```python
from build123d import *

# Parameters (mm, degrees)
F1_DEPTH      = 50.8
F1_DEPTH_BACK = 50.8


with BuildPart() as f1:
    # F0 (on Right) → F1 (new body, two sides)
    with BuildSketch(Plane.YZ) as f1_sk:
        with BuildLine():
            Line((-33.213852, 0), (0, 0))
            Line((0, 0), (39.494485, 0))
            Line((39.494485, 0), (39.494485, 0.787258))
            ThreePointArc((39.494485, 0.787258), (39.42009, 0.966864), (39.240485, 1.041258))
            Line((39.240485, 1.041258), (38.534891, 1.041258))
            ThreePointArc((38.534891, 1.041258), (38.355286, 1.115653), (38.280891, 1.295258))
            Line((38.280891, 1.295258), (38.280891, 1.323207))
            ThreePointArc((38.280891, 1.323207), (38.206496, 1.502813), (38.026891, 1.577207))
            Line((38.026891, 1.577207), (36.921442, 1.577207))
            ThreePointArc((36.921442, 1.577207), (36.739611, 1.653856), (36.667521, 1.837542))
            Line((36.667521, 1.837542), (36.67292, 2.053964))
            Line((36.67292, 2.053964), (36.67292, 10.407829))
            ThreePointArc((36.67292, 10.407829), (36.52413, 10.767039), (36.16492, 10.915829))
            Line((36.16492, 10.915829), (35.66636, 10.915829))
            ThreePointArc((35.66636, 10.915829), (35.529192, 10.956051), (35.435466, 11.063979))
            Line((35.435466, 11.063979), (34.805344, 12.438487))
            ThreePointArc((34.805344, 12.438487), (34.711619, 12.546415), (34.57445, 12.586637))
            Line((34.57445, 12.586637), (33.903744, 12.586637))
            ThreePointArc((33.903744, 12.586637), (33.752842, 12.536952), (33.660976, 12.407335))
            Line((33.660976, 12.407335), (32.40961, 8.340397))
            ThreePointArc((32.40961, 8.340397), (32.317744, 8.21078), (32.166843, 8.161095))
            Line((32.166843, 8.161095), (28.181681, 8.161095))
            Line((28.181681, 8.161095), (28.181681, 8.340397))
            Line((28.181681, 8.340397), (27.995555, 8.340397))
            Line((27.995555, 8.340397), (27.995555, 8.161095))
            Line((27.995555, 8.161095), (24.103897, 8.161095))
            Line((24.103897, 8.161095), (24.103897, 8.339632))
            Line((24.103897, 8.339632), (23.922047, 8.339632))
            Line((23.922047, 8.339632), (23.922047, 8.161095))
            Line((23.922047, 8.161095), (20.075496, 8.161095))
            Line((20.075496, 8.161095), (20.075496, 8.348511))
            Line((20.075496, 8.348511), (19.897439, 8.348511))
            Line((19.897439, 8.348511), (19.897439, 8.161095))
            Line((19.897439, 8.161095), (16.041223, 8.161095))
            Line((16.041223, 8.161095), (16.041223, 8.341497))
            Line((16.041223, 8.341497), (15.859049, 8.341497))
            Line((15.859049, 8.341497), (15.859049, 8.161095))
            Line((15.859049, 8.161095), (11.9808, 8.161095))
            Line((11.9808, 8.161095), (11.9808, 8.331576))
            Line((11.9808, 8.331576), (11.798942, 8.331576))
            Line((11.798942, 8.331576), (11.798942, 8.161095))
            Line((11.798942, 8.161095), (7.925448, 8.161095))
            Line((7.925448, 8.161095), (7.925448, 8.35035))
            Line((7.925448, 8.35035), (7.742784, 8.35035))
            Line((7.742784, 8.35035), (7.742784, 8.161095))
            Line((7.742784, 8.161095), (3.581181, 8.161095))
            ThreePointArc((3.581181, 8.161095), (3.444013, 8.201317), (3.350287, 8.309245))
            Line((3.350287, 8.309245), (1.457299, 12.438487))
            ThreePointArc((1.457299, 12.438487), (1.363573, 12.546415), (1.226405, 12.586637))
            Line((1.226405, 12.586637), (0, 12.586637))
            Line((0, 12.586637), (-1.226405, 12.586637))
            ThreePointArc((-1.226405, 12.586637), (-1.363573, 12.546415), (-1.457299, 12.438487))
            Line((-1.457299, 12.438487), (-3.350287, 8.309245))
            ThreePointArc((-3.350287, 8.309245), (-3.444013, 8.201317), (-3.581181, 8.161095))
            Line((-3.581181, 8.161095), (-7.742784, 8.161095))
            Line((-7.742784, 8.161095), (-7.742784, 8.35035))
            Line((-7.742784, 8.35035), (-7.925448, 8.35035))
            Line((-7.925448, 8.35035), (-7.925448, 8.161095))
            Line((-7.925448, 8.161095), (-11.798942, 8.161095))
            Line((-11.798942, 8.161095), (-11.798942, 8.331576))
            Line((-11.798942, 8.331576), (-11.9808, 8.331576))
            Line((-11.9808, 8.331576), (-11.9808, 8.161095))
            Line((-11.9808, 8.161095), (-15.859049, 8.161095))
            Line((-15.859049, 8.161095), (-15.859049, 8.341497))
            Line((-15.859049, 8.341497), (-16.041223, 8.341497))
            Line((-16.041223, 8.341497), (-16.041223, 8.161095))
            Line((-16.041223, 8.161095), (-19.897439, 8.161095))
            Line((-19.897439, 8.161095), (-19.897439, 8.348511))
            Line((-19.897439, 8.348511), (-20.075496, 8.348511))
            Line((-20.075496, 8.348511), (-20.075496, 8.161095))
            Line((-20.075496, 8.161095), (-23.922047, 8.161095))
            Line((-23.922047, 8.161095), (-23.922047, 8.339632))
            Line((-23.922047, 8.339632), (-24.103897, 8.339632))
            Line((-24.103897, 8.339632), (-24.103897, 8.161095))
            Line((-24.103897, 8.161095), (-27.995555, 8.161095))
            Line((-27.995555, 8.161095), (-27.995555, 8.340397))
            Line((-27.995555, 8.340397), (-28.181681, 8.340397))
            Line((-28.181681, 8.340397), (-28.181681, 8.161095))
            Line((-28.181681, 8.161095), (-32.166843, 8.161095))
            ThreePointArc((-32.166843, 8.161095), (-32.317744, 8.21078), (-32.40961, 8.340397))
            Line((-32.40961, 8.340397), (-33.660976, 12.407335))
            ThreePointArc((-33.660976, 12.407335), (-33.752842, 12.536952), (-33.903744, 12.586637))
            Line((-33.903744, 12.586637), (-34.57445, 12.586637))
            ThreePointArc((-34.57445, 12.586637), (-34.711619, 12.546415), (-34.805344, 12.438487))
            Line((-34.805344, 12.438487), (-35.435466, 11.063979))
            ThreePointArc((-35.435466, 11.063979), (-35.529192, 10.956051), (-35.66636, 10.915829))
            Line((-35.66636, 10.915829), (-36.16492, 10.915829))
            ThreePointArc((-36.16492, 10.915829), (-36.52413, 10.767039), (-36.67292, 10.407829))
            Line((-36.67292, 10.407829), (-36.67292, 2.053964))
            ThreePointArc((-36.67292, 2.053964), (-36.52413, 1.694754), (-36.16492, 1.545964))
            Line((-36.16492, 1.545964), (-34.873612, 1.545964))
            ThreePointArc((-34.873612, 1.545964), (-34.694007, 1.47157), (-34.619612, 1.291964))
            Line((-34.619612, 1.291964), (-34.619612, 1.104801))
            ThreePointArc((-34.619612, 1.104801), (-34.545217, 0.925196), (-34.365612, 0.850801))
            Line((-34.365612, 0.850801), (-33.721852, 0.850801))
            ThreePointArc((-33.721852, 0.850801), (-33.542246, 0.776406), (-33.467852, 0.596801))
            Line((-33.467852, 0.596801), (-33.467852, 0.254))
            ThreePointArc((-33.467852, 0.254), (-33.393457, 0.074395), (-33.213852, 0))
        make_face()
    extrude(amount=F1_DEPTH)
    extrude(f1_sk.sketch, amount=-F1_DEPTH_BACK)


solid = f1.part
```
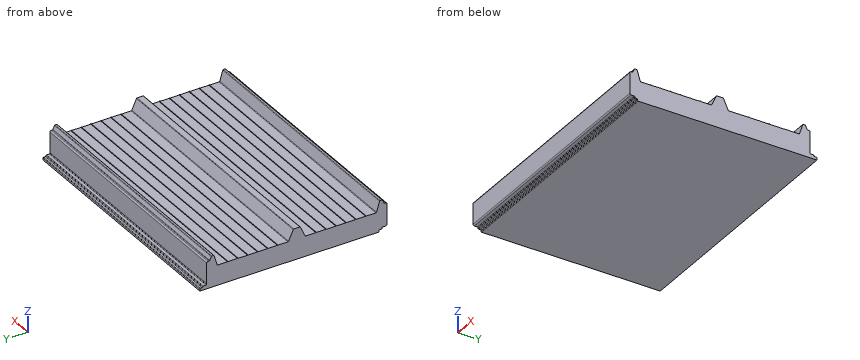
Input: part model. Units: mm. Frame: model coordinates. Coordinates: 2 decimals unless noted, no trailing zeros. Write each loop counter-clockwise with the first axis right and the second up, starting at its lowest first coordinate (ties: lowest second). Pieces come first, ordered by that corner, then holes. Notation, with made-up numbers: M -28,59.25 L -3,59.25 A16 ccw -3,85.25 Z; hole C 42.25,86 d5. An arc over 180 degrees is marked long. Use one line per item in the form item = value.
Q1. Material intervals for probe 1 along Y at (x, z) = (5.5, 11.5); probe 2 along Y at (x, z) = (-36.5, 11.25); probe 3 along Z at (x, y) = (34, -29), sorted ascending. Write a range as from..to.
Answer below:
probe_1 = -35.24..-33.38, -1.89..1.89, 33.38..35.24
probe_2 = -35.35..-33.3, -2..2, 33.3..35.35
probe_3 = 0..8.16
Q2. First-contact query: pin 1 (1.2 mm diameter, centred on x = -1.5, y = -10, fed in from +Z); pin 2 (0.6 mm diameter, centred on x = 13, y = 39, fed in from +Z); pin 3 (4.5 mm diameter, centred on x = -2.5, y = 6.5, fed in from +Z). Flat tips, straight axial feed; report the tip coordinate or a pass-through.
Answer below:
pin_1 = 8.16
pin_2 = 1.04
pin_3 = 8.35
Q3. Section A-A (z = 3.75). Return loops of the section in (x, y), plus the area to 3 significant figures.
Answer below:
outline = M -50.8,-36.67 L 50.8,-36.67 L 50.8,36.67 L -50.8,36.67 Z
area = 7,450 mm²
Q4. Section B-B (y = -22.5). Return loops of the section in (x, z).
Answer below:
outline = M -50.8,0 L 50.8,0 L 50.8,8.16 L -50.8,8.16 Z
